Can you work these out from the model? Positions are in its coordinate system, mm. Coordinates: 2 decimals unless noted, no trailing zeros. Order: outer loops, then holes, each group sorted by start corner. A loop starts at its lowest first (then second) coordinate and runs counter-clockwise, first axis right, second up.
```python
from build123d import *

# Parameters (mm, degrees)
SKETCH1_R          = 6.25
BASE_EXTRUDE_DEPTH = 10


with BuildPart() as part:
    # Sketch1 → Base-Extrude (new body)
    with BuildSketch(Plane.XY):
        with BuildLine():
            Line((29.785193593, -23.187206185), (54.059480558, -0.238916618))
            Line((54.059480558, -0.238916618), (54.059480558, 22.705666265))
            Line((54.059480558, 22.705666265), (11.211177394, 22.705666265))
            Line((11.211177394, 22.705666265), (11.211177394, -15.186351603))
            ThreePointArc((11.211177394, -15.186351603), (17.865606506, -25.298321636), (29.785193593, -23.187206185))
        make_face()
        with Locations((22.221390463, -15.186351603)):
            Circle(SKETCH1_R, mode=Mode.SUBTRACT)
        with Locations((39.837339904, 3.704441374)):
            Circle(SKETCH1_R, mode=Mode.SUBTRACT)
    extrude(amount=-BASE_EXTRUDE_DEPTH)


solid = part.part
```
1. Imagine slicing it at C-C on z = -2.5. Please give me the cut outline in (x, y), then the cut area to 3 significant figures.
Completed:
outline: (11.21, -15.19) arc R11.01 ccw to (29.79, -23.19) - (54.06, -0.24) - (54.06, 22.71) - (11.21, 22.71) - close; hole circle Ø12.5 at (22.22, -15.19); hole circle Ø12.5 at (39.84, 3.7)
area: 1,470 mm2
2. Imagine slicing it at B-B on y = -17.5. Please give me the cut outline in (x, z).
Completed:
outline: (11.46, -10) - (16.42, -10) - (16.42, 0) - (11.46, 0) - close; (28.03, -10) - (35.8, -10) - (35.8, 0) - (28.03, 0) - close
3. Imagine slicing it at A-A on x = 40.5. Please give me the cut outline in (y, z).
Completed:
outline: (-13.06, -10) - (-2.51, -10) - (-2.51, 0) - (-13.06, 0) - close; (9.92, -10) - (22.71, -10) - (22.71, 0) - (9.92, 0) - close
4. Imagine slicing it at D-D on x = 31.5. Please give me the cut outline in (y, z), then the cut area to 3 significant figures.
Completed:
outline: (-21.57, -10) - (22.71, -10) - (22.71, 0) - (-21.57, 0) - close
area: 443 mm2
5. Please list where these lines run through material, in increasing order: probe 1 along Y at (x, z) = (44.5, -6.75); probe 2 along Y at (x, z) = (17, -4); probe 3 along X at (y, z) = (-16, -8).
Completed:
probe 1: y = -9.28 to -0.46, 7.87 to 22.71
probe 2: y = -24.88 to -18.62, -11.75 to 22.71
probe 3: x = 11.24 to 16.02, 28.42 to 37.39
6. I'm going to push flat-ended pins straight in: pin 1 (6 mm diameter, centred on x = 43.5, z = -3, fed in from -Y); pin 2 (11 mm diameter, centred on x = 22.22, y = -15.19, fed in from +Z); pin 3 (20 mm diameter, centred on x = 39.84, y = 3.7, fed in from +Z); pin 4 (2 mm diameter, centred on y = -8, z = -7.5, fed in from +X). Where does each tip first touch, or does it pass through?
Completed:
pin 1: stops at y = -13.06
pin 2: passes through
pin 3: stops at z = 0
pin 4: stops at x = 46.91
